The figure shows three views and two pictorial views of one solid part (mm, origin at its lowest corner). Answer the questions. A direction names the side the tool comes from. Give positions to 0.01 mm unless a question says otherwise; leave off trailing zeros. Loops run counter-clockwise (first coordinate to the right, second up) from the corner with the lowest first, then second, coordinate; pieces in that order, holes last. Notation, with made-up numbers: M 12,59 L 58,59 A16 ccw 58,70 Z; hole C 51.25,54 d7. An arc over 180 degrees is marked long. Write item = value, one per line. Start each with the question number.
1. Section A-A on y = 37.5 is taken. Determine the outline of the cut face in (x, z).
2. Section D-D on x = 23.5 is taken. Determine the outline of the cut face in (y, z) (1 decimal).
3. Section B-B on x = 18 is taken. Determine the outline of the cut face in (y, z).
4. Consider L1, parallel to Y at x = 20.5, z = 1.5; L2, parallel to Z at x = 30, y = 13. Determine where each line is inside the solid, lowest interval first. Write a range as [from, to].
5. Flat-ended cylindrical pins translate along their axes: pin 1 Ø1 at (x, y) = (8, 29) entering from +Z; pin 2 Ø1.5 at (x, z) = (29.5, 45) entering from +Y. Find the tip coordinate at first contact, or state that the pin passes through.
6. For the marked faces 1 and 2, determine the directions among +Z, -Z, +X, -X, +Y, -Y from which every point of the face is accessible in a straight line to the end or side of a thin tool.
7. Section C-C on y = 20 is taken. Determine the outline of the cut face in (x, z), plus the area to 3 significant figures.
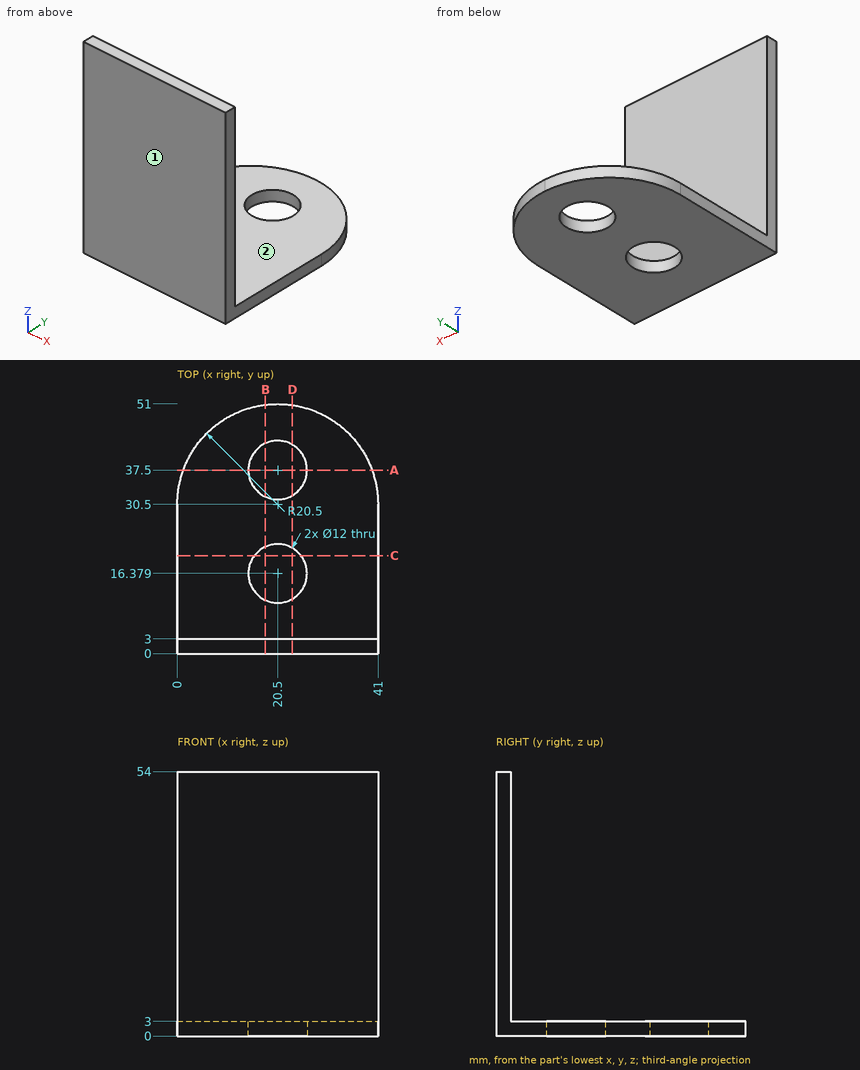
Verdict:
q1.outline = M 1.23,0 L 14.5,0 L 14.5,3 L 1.23,3 Z; M 26.5,0 L 39.77,0 L 39.77,3 L 26.5,3 Z
q2.outline = M 0,0 L 11.2,0 L 11.2,3 L 3,3 L 3,54 L 0,54 Z; M 21.6,0 L 32.3,0 L 32.3,3 L 21.6,3 Z; M 42.7,0 L 50.8,0 L 50.8,3 L 42.7,3 Z
q3.outline = M 0,0 L 10.92,0 L 10.92,3 L 3,3 L 3,54 L 0,54 Z; M 21.83,0 L 32.05,0 L 32.05,3 L 21.83,3 Z; M 42.95,0 L 50.85,0 L 50.85,3 L 42.95,3 Z
q4.L1 = [0, 10.38], [22.38, 31.5], [43.5, 51]
q4.L2 = [0, 3]
q5.pin_1 = 3
q5.pin_2 = 3
q6.face_1 = +Z, -Z, +X, -X, -Y
q6.face_2 = +Z, +X, -X, +Y
q7.outline = M 0,0 L 15.72,0 L 15.72,3 L 0,3 Z; M 25.28,0 L 41,0 L 41,3 L 25.28,3 Z
q7.area = 94.3 mm2
